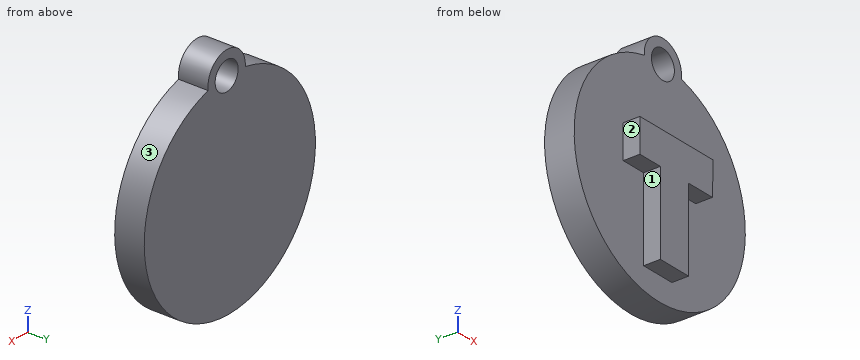
from build123d import *

# Parameters (mm, degrees)
F0_R     = 2.306081
F1_DEPTH = 4.7625
F2_W     = 5.668672
F2_H     = 13.29764
F3_DEPTH = 2.6924


with BuildPart() as f1:
    # F0 (on Front) → F1 (new body)
    with BuildSketch(Plane.XZ):
        with BuildLine():
            ThreePointArc((-3.100331, 16.875266), (-0.634898, -17.145949), (4.339878, 16.599763))
            ThreePointArc((4.339878, 16.599763), (0.773477, 20.888408), (-3.100331, 16.875266))
        make_face()
        with Locations((0.634898, 17.145949)):
            Circle(F0_R, mode=Mode.SUBTRACT)
    extrude(amount=F1_DEPTH)

    # F2 (on face) → F3 (join)
    with BuildSketch(Plane.XZ.offset(4.7625)):
        Polygon((-7.326433, 5.411912), (-7.326433, 0), (-3.225957, 0), (2.442715, 0), (6.360534, 0), (7.207565, 0), (7.381472, 5.411912), align=None)
        with Locations((-0.391621, -6.64882)):
            Rectangle(F2_W, F2_H)
    extrude(amount=F3_DEPTH)


solid = f1.part
Verification items for the finished model (mm, model axes). Face numbers are marked on the shaded views. A direction names the side the tool comes from. Give positions to 0.01 mm unless a question says otherwise; leave off trailing zeros. Order: outer loops, then holes, each group sorted by start corner. A loop starts at its lowest first (then second) coordinate and runs counter-clockwise, first axis right, second up. Notation, with made-up numbers: M 16.5,28 L 61.5,28 A20 cw 61.5,35 Z; hole C 85.5,-22.5 d1. An arc over 180 degrees is marked long. Use one line per item in the form item = value. Start each with the question number.
Q1. Section check C-C (y = -6). Enter the section's corners in (x, z).
Q2. Section check B-B (z = 18). Enter the section's corners in (x, y).
Q3. Access from +Z, -Z, +X, -X, +Y, -Y to the whole of each face (thin tool, end or side, straight path). Record for the marked faces 1, 2 and 3.
Q4. Go/stop test with flat-tipped pins: pin 1 Ø1.5 at (y, z) = (-2.5, -8.5) entering from -X; pin 2 Ø5 at (x, z) = (8.5, 10.5) entering from +Y; pin 3 Ø3 at (y, z) = (-6.5, -7.5) entering from -X; pin 4 Ø3 at (x, y) = (-5, -6) entering from -Z. Record where each tip stops, or that it passes through.
Q5. Section check A-A (x = 1.5). Enter the section's corners in (y, z), then the cut area to 3 significant figures.
Q6. Section check D-D (z = -7.5). Enter the section's corners in (x, y), then the cut area to 3 significant figures.
Q7. Scan lines: line 1 along Z through (x, y) = (0.5, -2); line 2 along X through (y, z) = (-4.5, 17); line 3 along Y through (x, z) = (13.5, -9). Record each from-to range of solid material in increasing order. Write a range as [from, to].
Evaluation:
q1.outline = M -7.33,0 L -3.23,0 L -3.23,-13.3 L 2.44,-13.3 L 2.44,0 L 7.21,0 L 7.38,5.41 L -7.33,5.41 Z
q2.outline = M -3.01,-4.76 L -1.51,-4.76 L -1.51,0 L -3.01,0 Z; M 2.78,-4.76 L 4.28,-4.76 L 4.28,0 L 2.78,0 Z
q3.face_1 = -Z, -X, -Y
q3.face_2 = +Z, -Z, -X, -Y
q3.face_3 = +Y, -Y
q4.pin_1 = -15.31
q4.pin_2 = 0
q4.pin_3 = -3.23
q4.pin_4 = -16.65
q5.outline = M -7.45,-13.3 L -4.76,-13.3 L -4.76,-17.09 L 0,-17.09 L 0,15.01 L -4.76,15.01 L -4.76,5.41 L -7.45,5.41 Z; M -4.76,19.28 L 0,19.28 L 0,20.79 L -4.76,20.79 Z
q5.area = 210 mm2
q6.outline = M -15.43,-4.76 L -3.23,-4.76 L -3.23,-7.45 L 2.44,-7.45 L 2.44,-4.76 L 15.43,-4.76 L 15.43,0 L -15.43,0 Z
q6.area = 162 mm2
q7.line_1 = [-17.15, 14.84], [19.45, 20.89]
q7.line_2 = [-3.11, -1.67], [2.94, 4.38]
q7.line_3 = [-4.76, 0]
